from build123d import *

# Parameters (mm, degrees)
BOSS_EXTRUDE1_DEPTH = 0.45
FILLET1_R           = 0.15


with BuildPart() as part:
    # Sketch1 → Boss-Extrude1 (new, symmetric)
    with BuildSketch(Plane(origin=(0, 0, 0), x_dir=(0, 0, -1), z_dir=(1, 0, 0))):
        Polygon((0, 0), (2.552076819, 0.45), (0, 0.9), (-10, 0.9), (-10, 0), align=None)
    extrude(amount=BOSS_EXTRUDE1_DEPTH, both=True)

    # Fillet1
    fillet1_edges = [part.edges().sort_by_distance(p)[0] for p in [
        (0, 0.45, -2.552076819),
    ]]
    fillet(fillet1_edges, radius=FILLET1_R)


solid = part.part
Model file for the job. Use its own axes, mm. Give positions to 0.01 mm unless a question says otherwise; leave off trailing zeros. Write each loop counter-clockwise with the first axis right and the second up, starting at its lowest first coordinate (ties: lowest second). Pieces come first, ordered by that corner, then holes. Notation, with made-up numbers: (64, 69) - (97, 69) arc R11 ccw to (97, 88) - close; hole circle Ø9 at (26, 23.25). An arc over 180 degrees is marked (long way). Answer as CSV lines item,"result".
1. Band-saw the part on B-B (y = 0.2). Write the cut outline in (x, z).
Responses:
outline,"(-0.45, -1.13) - (0.45, -1.13) - (0.45, 10) - (-0.45, 10) - close"
2. Band-saw the part on A-A (x = 0.2). Write the cut outline in (y, z).
Responses:
outline,"(0, 0) - (0.3, -1.71) arc R0.15 ccw to (0.6, -1.71) - (0.9, 0) - (0.9, 10) - (0, 10) - close"
3. Band-saw the part on C-C (y = 0.75). Write the cut outline in (x, z), and give its area (3 significant figures).
Responses:
outline,"(-0.45, -0.85) - (0.45, -0.85) - (0.45, 10) - (-0.45, 10) - close"
area,"9.77 mm2"
4. Drill centre lines: L1, parallel to Z at x = -0.15, y = 0.4; L2, parallel to Y at x = 0.3, z = -0.5. Where is each one in solid material? Low to high. Write a range as [from, to].
Responses:
L1,"z = [-1.83, 10]"
L2,"y = [0.09, 0.81]"
